Check sheet for the modelled part. Datum: model origin and axes. Units: mm. Face numbers are marked on the shaded views. A direction names the side the tool comes from. Round coordinates to 2 decimals unless told otherwise and drop trailing zeros. Write each loop counter-clockwise with the first axis right and the second up, starting at its lowest first coordinate (ties: lowest second). Pieces come first, ordered by that corner, then holes.
Item 1: Go/stop test with flat-tipped pins: pin 1 Ø1.1 at (x, y) = (0, 3.5) entering from -Z; pin 2 Ø1.2 at (x, z) = (4, 2.5) entering from +Y; pin 3 Ø0.7 at (x, z) = (-3.5, 1) entering from +Y; pin 4 Ø2 at (x, z) = (-0.5, 0.5) entering from +Y. Record where each tip stops, or that it passes through.
Item 2: Tool access check on the marked faces 1, 2 and 3. Record the directions out of +Z, -Z, +X, -X, +Y, -Y that give a thin tool (end or side, any length) a straight path to the whole face; none if there is none.
Item 3: Release check for a two-part mould opening along X. For the marked faces 4, 5 and 6 record: +X half, -X half, draft (parallel to the pull), parting line (faces both ways), or undercut.
Item 4: Material ranges on line 1 (Z direction, x = 0, y = 1.9); line 2 (Y direction, x = 4.5, z = 1); line 3 (X direction, y = 4.8, z = -1.5), recorded low to high.
Item 5: Cross-section at A-A on y = 1.15. Enter the section's corners in (x, z), plus the area to 3 significant figures.
from build123d import *

# Parameters (mm, degrees)
SKETCH1_R               = 5.5
BOSS_EXTRUDE1_DEPTH     = 1.5
CHAMFER1_SIZE           = 0.6
CHAMFER1_SIZE2          = 0.856888804
BOSS_EXTRUDE2_DEPTH     = 3.5
SKETCH3_R               = 4.021052248
BOSS_EXTRUDE3_DEPTH     = 1
SKETCH5_R               = 2.121052248
CUT_EXTRUDE1_DEPTH      = 0.6
FILLET1_R               = 0.9
CUT_EXTRUDE2_DEPTH      = 10.468896451
CUT_EXTRUDE2_DEPTH_BACK = 10.468896451
SKETCH6_R               = 2


with BuildPart() as part:
    # Sketch1 → Boss-Extrude1 (new body)
    with BuildSketch(Plane(origin=(0, 0, 0), x_dir=(1, 0, 0), z_dir=(0, 1, 0))):
        with Locations(Location((0, 0, 0), (0, 0, 270))):
            Circle(SKETCH1_R)
    extrude(amount=BOSS_EXTRUDE1_DEPTH)

    # Chamfer1
    chamfer1_edges = [part.edges().sort_by_distance(p)[0] for p in [
        (0, 1.5, -5.5),
    ]]
    chamfer1_side = [part.faces().sort_by_distance(p)[0] for p in [
        (0, 0.75, -5.5),
    ]]
    chamfer(chamfer1_edges, length=CHAMFER1_SIZE, length2=CHAMFER1_SIZE2, reference=chamfer1_side[0])

    # Sketch2 → Boss-Extrude2 (add)
    with BuildSketch(Plane(origin=(0, 1.5, 0), x_dir=(1, 0, 0), z_dir=(0, 1, 0))):
        Polygon((4.643111196, 0), (2.321555598, 4.021052248), (-2.321555598, 4.021052248), (-4.643111196, 0), (-2.321555598, -4.021052248), (2.321555598, -4.021052248), align=None)
    extrude(amount=BOSS_EXTRUDE2_DEPTH)

    # Sketch3 → Boss-Extrude3 (add)
    with BuildSketch(Plane(origin=(0, 5, 0), x_dir=(1, 0, 0), z_dir=(0, 1, 0))):
        with Locations(Location((0, 0, 0), (0, 0, 270))):
            Circle(SKETCH3_R)
    extrude(amount=BOSS_EXTRUDE3_DEPTH)

    # Sketch4 → Cut-Revolve1 (revolve, cut)
    with BuildSketch(Plane.XY, mode=Mode.PRIVATE) as cut_revolve1_sk:
        with BuildLine():
            Line((6.63749378, 2.793667141), (6.63749378, 7.491604904))
            Line((6.63749378, 7.491604904), (3.021052248, 7.491604904))
            Line((3.021052248, 7.491604904), (3.021052248, 6))
            ThreePointArc((3.021052248, 6), (3.728159029, 5.707106781), (4.021052248, 5))
            ThreePointArc((4.021052248, 5), (5.485320065, 4.081886331), (6.63749378, 2.793667141))
        make_face()
    revolve(cut_revolve1_sk.sketch.rotate(Axis((0, 6, 0), (0, 1, 0)), 60), axis=Axis((0, 6, 0), (0, 1, 0)), mode=Mode.SUBTRACT)

    # Sketch5 → Cut-Extrude1 (cut)
    with BuildSketch(Plane(origin=(0, 6, 0), x_dir=(1, 0, 0), z_dir=(0, 1, 0))):
        with Locations(Location((0, 0, 0), (0, 0, 270))):
            Circle(SKETCH5_R)
    extrude(amount=-CUT_EXTRUDE1_DEPTH, mode=Mode.SUBTRACT)

    # Fillet1
    # the kernel refuses this fillet: 0.9 mm, written as the material it takes off along each edge
    with BuildSketch(Plane(origin=(0, 6, 0), x_dir=(0, 0, 1), z_dir=(-1, 0, 0))) as fillet1_piece_1:
        with BuildLine():
            CenterArc((2.969580386, -0.9), FILLET1_R, 90, 70.528779366)
            Line((2.121052248, -0.6), (2.104081686, -0.594))
            ThreePointArc((2.104081686, -0.594), (2.103052248, -0.3), (2.103052248, 0))
            Line((2.103052248, 0), (2.121052248, 0.018))
            Line((2.121052248, 0.018), (2.969580386, 0.018))
            Line((2.969580386, 0.018), (2.969580386, 0))
        make_face()
    revolve(axis=Axis((0, 6, 0), (0, 1, 0)), mode=Mode.SUBTRACT)

    # Sketch6 → Cut-Extrude2 (cut, two sides: drawn at the far end of the back side and taken through both)
    with BuildSketch(Plane(origin=(0, 5.4, 0), x_dir=(1, 0, 0), z_dir=(0, 1, 0)).offset(-CUT_EXTRUDE2_DEPTH_BACK)):
        with Locations(Location((0, 0, 0), (0, 0, 270))):
            Circle(SKETCH6_R)
    extrude(amount=CUT_EXTRUDE2_DEPTH + CUT_EXTRUDE2_DEPTH_BACK, mode=Mode.SUBTRACT)


solid = part.part
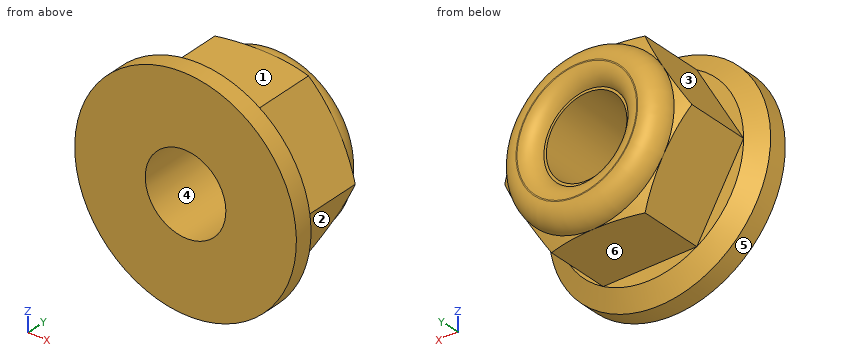
Response values:
1. pin 1: stops at z = -4.02
1. pin 2: stops at y = 1.5
1. pin 3: stops at y = 5.96
1. pin 4: passes through
2. face 1: +Z, +X, -X, +Y
2. face 2: -Z, +X, +Y
2. face 3: +Z, -X, +Y
3. face 4: undercut
3. face 5: parting line
3. face 6: draft
4. line 1: z = -4.02 to -2, 2 to 4.02
4. line 2: y = 0 to 1.5
4. line 3: x = -3.78 to -1.32, 1.32 to 3.78
5. outline: circle Ø10.29 at (0, 0); hole circle Ø4 at (0, 0)
5. area: 70.5 mm2
